```python
from build123d import *

# Parameters (mm, degrees)
SKETCH007_R   = 18.25
SKETCH007_R_2 = 2.5
PAD002_DEPTH  = 5
POCKET_DEPTH  = 2.75
CHAMFER_SIZE  = 1


with BuildPart() as part:
    # Sketch007 → Pad002 (new body, symmetric)
    with BuildSketch(Plane.XY):
        with BuildLine():
            ThreePointArc((0, 22.5), (-22.5, 0), (0, -22.5))
            Line((0, -22.5), (46, -22.5))
            ThreePointArc((46, -22.5), (68.5, 0), (46, 22.5))
            Line((0, 22.5), (46, 22.5))
        make_face()
        Circle(SKETCH007_R, mode=Mode.SUBTRACT)
        with Locations((46, 0)):
            Circle(SKETCH007_R, mode=Mode.SUBTRACT)
        with Locations((23, 16.2)):
            Circle(SKETCH007_R_2, mode=Mode.SUBTRACT)
        with Locations((23, -16.2)):
            Circle(SKETCH007_R_2, mode=Mode.SUBTRACT)
    extrude(amount=PAD002_DEPTH, both=True)

    # Sketch069 → Pocket (cut, symmetric)
    with BuildSketch(Plane.XY):
        with BuildLine():
            Line((29.25, 55.400131), (29.25, 16.2))
            ThreePointArc((16.75, 16.2), (23, 9.95), (29.25, 16.2))
            Line((16.75, 16.2), (16.75, 45.38327))
            Line((16.75, 45.38327), (-33.812714, 45.38327))
            Line((-33.812714, 45.38327), (-33.812714, -45.794624))
            Line((-33.812714, -45.794624), (16.75, -45.794624))
            Line((16.75, -16.2), (16.75, -45.794624))
            ThreePointArc((29.25, -16.2), (23, -9.95), (16.75, -16.2))
            Line((29.25, -53.709297), (29.25, -16.2))
            Line((29.25, -53.709297), (-45.873169, -53.709297))
            Line((-45.873169, -53.709297), (-45.873169, 55.400131))
            Line((-45.873169, 55.400131), (29.25, 55.400131))
        make_face()
    extrude(amount=POCKET_DEPTH, both=True, mode=Mode.SUBTRACT)

    # Chamfer
    chamfer_edges = [part.edges().sort_by_distance(p)[0] for p in [
        (20.5, 16.2, 5),
        (20.5, -16.2, 5),
    ]]
    chamfer(chamfer_edges, length=CHAMFER_SIZE)


solid = part.part
```
Here's how the part is built. I have some questions about the finished solid (model axes, mm). A direction names the side the tool comes from. Give positions to 0.01 mm unless a question says otherwise; leave off trailing zeros. Loops run counter-clockwise (first coordinate to the right, second up) from the corner with the lowest first, then second, coordinate; pieces in that order, holes last. Notation, with made-up numbers: (30.25, -5.75) -> (36.25, -5.75) arc R33 ccw to (36.25, 30.25) -> close; hole circle Ø7 at (10, 77.25). An arc over 180 degrees is marked (long way). Use one line per item in the form item = value. Start each with the question number.
1) Imagine slicing it at C-C (z = -0.75). Please give me the cut outline in (x, y), then the cut area to 3 significant figures.
2) Which directions (+Z, -Z, +X, -X, +Y, -Y) give clear straight access to the entire face, cutting with the end or side of a thin tool? Please do faces 3 (the face through (23.14, -9.95, 0.04)), 4 (the face through (16.75, 19, 0)), 5 (the face through (-3.956, -17.816, -0.07)).
3) For P1, Ø6.5, axis at x = 24.5, y = 15.5, coming from the -Z side; P2, Ø5, axis at y = -7.5, z = 2.5, coming from the +X side; P3, Ø1.6, axis at y = 20.5, z = 0, coming from the -X side; P4, Ø5, axis at y = -8, z = -3.5, coming from the -X side, each with a flat end and sliding along its axis, tell me the tip position at first contact or that it passes through.
4) Thinking about a two-plate mould opening in Z: for faces 1 (the face through (22.86, 9.95, 0.04)), 2 (the face through (23, 22.5, 3)), which applies, +Z half, -Z half, draft (parallel to the pull), parting line (faces both ways), or undercut?
5) Imagine slicing it at B-B (x = 23). Count the separate pieces of the cut face and the enclosed holes in it, then the cut area to 3 significant figures.
6) Imagine slicing it at A-A (y = 0). Please give me the cut outline in (x, z), then the cut area to 3 significant figures.
7) Please list where these lines run through material, in increasing order: line 1 along Y through (x, z) = (23, -4.25); line 2 along X through (y, z) = (-1.5, 0); line 3 along X through (y, z) = (-9.5, -4.5).
8) Imagine slicing it at D-D (x = 47). Please give me the cut outline in (y, z), then the cut area to 3 significant figures.
Check values:
q1.outline = (0, -22.5) -> (16.75, -22.5) -> (16.75, -16.2) arc R6.25 cw to (29.25, -16.2) -> (29.25, -22.5) -> (46, -22.5) arc R22.5 ccw to (46, 22.5) -> (29.25, 22.5) -> (29.25, 16.2) arc R6.25 cw to (16.75, 16.2) -> (16.75, 22.5) -> (0, 22.5) arc R22.5 ccw to start; hole circle Ø36.5 at (0, 0); hole circle Ø36.5 at (46, 0)
q1.area = 1,290 mm^2
q2.face_3 = -Y
q2.face_4 = +Y
q2.face_5 = +Z, -Z
q3.P1 = -5
q3.P2 = 67.94
q3.P3 = -10.87
q3.P4 = -21.82
q4.face_1 = undercut
q4.face_2 = draft
q5.separate_pieces = 5
q5.enclosed_holes = 0
q5.area = 265 mm^2
q6.outline = (-22.5, -5) -> (-18.25, -5) -> (-18.25, 5) -> (-22.5, 5) -> close; (18.25, -5) -> (27.75, -5) -> (27.75, 5) -> (18.25, 5) -> close; (64.25, -5) -> (68.5, -5) -> (68.5, 5) -> (64.25, 5) -> close
q6.area = 180 mm^2
q7.line_1 = -22.5 to -18.7, -13.7 to 13.7, 18.7 to 22.5
q7.line_2 = -22.45 to -18.19, 18.19 to 27.81, 64.19 to 68.45
q7.line_3 = -20.4 to -15.58, 15.58 to 30.42, 61.58 to 66.4
q8.outline = (-22.48, -5) -> (-18.22, -5) -> (-18.22, 5) -> (-22.48, 5) -> close; (18.22, -5) -> (22.48, -5) -> (22.48, 5) -> (18.22, 5) -> close
q8.area = 85.1 mm^2
